Part model, mm, in its own coordinate system. A direction names the side the tool comes from. Round coordinates to 2 decimals unless told otherwise and drop trailing zeros. Write each loop counter-clockwise with the first axis right and the second up, starting at its lowest first coordinate (ties: lowest second). Pieces come first, ordered by that corner, then holes. Notation, with made-up numbers: (20.5, 28) -> (33.5, 28) arc R17 ccw to (33.5, 61) -> close; hole circle Ø11 at (5, 42). An arc over 180 degrees is marked (long way). Use CSV: the item, a comma, the result in double quotes. Start each with the question number.
```python
from build123d import *


with BuildPart() as part:
    # Sweep1: sweep along a path in Sketch1
    with BuildLine(Plane.XY.offset(133.35)) as sweep1_path:
        Line((-784.071645386, -162.117385896), (-591.554631016, -51.243460213))
        Line((-591.554631016, -51.243460213), (-402.166018744, -22.095582214))
        Line((-402.166018744, -22.095582214), (-211.416027506, -7.512293336))
        Line((-211.416027506, -7.512293336), (-22.665229034, -1.270332507))
        Line((-22.665229034, -1.270332507), (166.165138103, -4.260913688))
        Line((166.165138103, -4.260913688), (357.125134769, -15.536328702))
        Line((357.125134769, -15.536328702), (546.775185731, -45.538131397))
        Line((546.775185731, -45.538131397), (733.483443068, -116.654162228))
    # Sketch2 → Sweep1 (sweep)
    with BuildSketch(Plane(origin=(0, 0, 0), x_dir=(0, 0, -1), z_dir=(1, 0, 0))):
        Polygon((-133.35, -1.638900587), (-128.752617541, -4.293200587), (-133.934217541, -13.267995051), (-138.5316, -10.613695051), align=None)
    sweep(path=sweep1_path.line, transition=Transition.RIGHT)


solid = part.part
```
1. Band-saw the part on B-B (z = 130.25). List the corners of the cut face in (x, y).
2. Drill centre lines: line 1 along Y through (x, z) = (478.5, 134.5); line 2 along Y through (x, z) = (84.5, 132.75); line 3 along Z through (x, y) = (261, -15). Where is each one in solid material? Low to high. Write a range as [from, to].
3. Band-saw the part on D-D (x = 419.5). List the corners of the cut face in (y, z).
4. Flat gauge pins, fed straight in: pin 1 (4 mm diameter, centred on y = -152, z = 134.5, fed in from +X); pin 2 (4 mm diameter, centred on x = -10, z = 135.5, fed in from +Y); pin 3 (5 mm diameter, centred on x = 382.5, y = -20, fed in from +Z). Where does each tip first touch, or does it go through?
5. Band-saw the part on A-A (y = -103). List the corners of the cut face in (x, z), then the cut area to 3 significant figures.
6. Pull direction X, two halves, no side cores. Call faces 4 (the flat face through (-494.175, -43.551, 131.378)), 5 (the flat face through (452.659, -35.099, 135.882)), 6 (the flat face through (-495.31, -37.8, 131.02)): released by +X, released by -X, zero draft, split by the parting line, or undercut.
7. Band-saw the part on C-C (x = -287.5). List the corners of the cut face in (y, z).
8. Which spindle directions (+Z, -Z, +X, -X, +Y, -Y) get a long thin tool onto all of the face, cutting with end or side? Do faces 1 (the flat face through (451.439, -40.865, 136.284)), 2 (the flat face through (639.935, -85.731, 135.885)), 3 (the flat face through (-304.813, -21.885, 131.379)). Say none if no direction does.
Answers below:
1,outline,"(-783.15, -163.66) -> (-781.38, -166.63) -> (-589.78, -56.29) -> (-401.56, -27.32) -> (-211.13, -12.76) -> (-22.62, -6.53) -> (165.97, -9.52) -> (356.56, -20.77) -> (545.41, -50.65) -> (731.69, -121.6) -> (732.87, -118.35) -> (546.31, -47.29) -> (356.93, -17.33) -> (166.1, -6.06) -> (-22.65, -3.07) -> (-211.32, -9.31) -> (-401.96, -23.88) -> (-590.95, -52.97) -> close"
2,line 1,"y = [-46.19, -36.76]"
2,line 2,"y = [-12.56, -3.32]"
2,line 3,"z = [130.18, 136.31]"
3,outline,"(-37.19, 133.93) -> (-28.1, 128.75) -> (-25.41, 133.35) -> (-34.5, 138.53) -> close"
4,pin 1,"stops at x = -739.86"
4,pin 2,"stops at y = -1.74"
4,pin 3,"stops at z = 135.04"
5,outline,"(-681.4, 133.35) -> (-676.09, 128.75) -> (-658.1, 133.93) -> (-663.42, 138.53) -> close; (664.94, 133.93) -> (690.15, 128.75) -> (697.61, 133.35) -> (672.4, 138.53) -> close"
5,area,"265 mm^2"
6,face 4,"undercut"
6,face 5,"released by +X"
6,face 6,"released by -X"
7,outline,"(-25, 133.93) -> (-16, 128.75) -> (-13.34, 133.35) -> (-22.34, 138.53) -> close"
8,face 1,"+Z, -Y"
8,face 2,"+Z, +X, +Y"
8,face 3,"-Z, -Y"
